from build123d import *

# Parameters (mm, degrees)
SKETCH1_W           = 19.8
SKETCH1_H           = 25
SKETCH1_R           = 1.15
BOSS_EXTRUDE1_DEPTH = 3
SKETCH2_W           = 19.8
SKETCH2_H           = 3
BOSS_EXTRUDE2_DEPTH = 26
CHAMFER1_SIZE       = 3
CUT_EXTRUDE1_DEPTH  = 15
CHAMFER2_SIZE       = 4
FILLET2_R           = 0.5


with BuildPart() as part:
    # Sketch1 → Boss-Extrude1 (new body)
    with BuildSketch(Plane.XY):
        with Locations((0, 1.287671233)):
            Rectangle(SKETCH1_W, SKETCH1_H)
        with Locations((-4.75, 10.787671233)):
            Circle(SKETCH1_R, mode=Mode.SUBTRACT)
        with Locations(Location((4.75, 10.787671233, 0), (0, 0, 180))):
            Circle(SKETCH1_R, mode=Mode.SUBTRACT)
    extrude(amount=BOSS_EXTRUDE1_DEPTH)

    # Sketch2 → Boss-Extrude2 (add)
    with BuildSketch(Plane.XY.offset(3)):
        with Locations((0, -9.712328767)):
            Rectangle(SKETCH2_W, SKETCH2_H)
    extrude(amount=BOSS_EXTRUDE2_DEPTH)

    # Chamfer1
    chamfer1_edges = [part.edges().sort_by_distance(p)[0] for p in [
        (0, -8.212328767, 3),
        (-9.9, 13.787671233, 1.5),
        (9.9, 13.787671233, 1.5),
    ]]
    chamfer(chamfer1_edges, length=CHAMFER1_SIZE)

    # Sketch4 → Cut-Extrude1 (cut)
    with BuildSketch(Plane(origin=(0, -8.212328767, 0), x_dir=(1, 0, 0), z_dir=(0, 1, 0))):
        with BuildLine():
            Line((2.647058824, -22.5), (2.647058824, -9.5))
            ThreePointArc((2.647058824, -9.5), (4.797058824, -7.35), (6.947058824, -9.5))
            Line((6.947058824, -9.5), (6.947058824, -22.5))
            ThreePointArc((6.947058824, -22.5), (4.797058824, -24.65), (2.647058824, -22.5))
        make_face()
        with BuildLine():
            Line((-2.647058824, -22.5), (-2.647058824, -9.5))
            ThreePointArc((-2.647058824, -9.5), (-4.797058824, -7.35), (-6.947058824, -9.5))
            Line((-6.947058824, -9.5), (-6.947058824, -22.5))
            ThreePointArc((-6.947058824, -22.5), (-4.797058824, -24.65), (-2.647058824, -22.5))
        make_face()
    extrude(amount=-CUT_EXTRUDE1_DEPTH, mode=Mode.SUBTRACT)

    # Chamfer2
    chamfer2_edges = [part.edges().sort_by_distance(p)[0] for p in [
        (-9.9, -9.712328767, 29),
        (9.9, -9.712328767, 29),
    ]]
    chamfer(chamfer2_edges, length=CHAMFER2_SIZE)

    # Fillet2
    fillet2_edges = [part.edges().sort_by_distance(p)[0] for p in [
        (-5.9, 10.787671233, 0),
        (5.9, 10.787671233, 0),
        (0, 13.787671233, 0),
        (0, 13.787671233, 3),
        (-6.9, 13.787671233, 1.5),
        (6.9, 13.787671233, 1.5),
        (-9.9, -0.212328767, 0),
        (-8.4, 12.287671233, 0),
        (8.4, 12.287671233, 0),
        (9.9, 2.787671233, 3),
        (9.9, 10.787671233, 1.5),
        (-9.9, 2.787671233, 3),
        (-8.4, 12.287671233, 3),
        (8.4, 12.287671233, 3),
        (-9.9, 10.787671233, 1.5),
        (-9.9, -6.712328767, 4.5),
        (9.9, -6.712328767, 4.5),
        (0, -11.212328767, 0),
        (9.9, -0.212328767, 0),
        (-5.9, -9.712328767, 29),
        (5.9, -9.712328767, 29),
        (9.9, -8.212328767, 15.5),
        (-9.9, -8.212328767, 15.5),
        (9.9, -11.212328767, 12.5),
        (9.9, -9.712328767, 25),
        (-9.9, -11.212328767, 12.5),
        (-9.9, -9.712328767, 25),
    ]]
    fillet(fillet2_edges, radius=FILLET2_R)


solid = part.part
The listing builds one solid part. Answer for the finished solid, in the listing's coordinates (mm). A direction names the side the tool comes from. Give positions to 0.01 mm unless a question says otherwise; leave off trailing zeros. Write each loop counter-clockwise with the first axis right and the second up, starting at its lowest first coordinate (ties: lowest second). Pieces come first, ordered by that corner, then holes. Notation, with made-up numbers: (-36.5, -2) -> (5.5, -2) arc R18 cw to (5.5, 18) -> close; hole circle Ø4 at (-19.75, -20.5). An arc over 180 degrees is marked (long way). Use a Markdown table: item, result.
(1) Determine the mould class of faces 1 (the flat face through (-2.647, -10, 16)), 2 (the flat face through (0, 13.788, 1)), 3 (the flat face through (-7.9, -9.7, 27)), 4 (the cylindrical face through (-4.84, -9.69, 24.65)) for opening direction Z: released by +Z, released by -Z, zero draft, split by the parting line, or undercut.
Return value:
| item | result |
|---|---|
| face 1 | undercut |
| face 2 | zero draft |
| face 3 | released by +Z |
| face 4 | undercut |
(2) Section B-B, the plane z = 15.75 is taken. Determine the outline of the cut face in (x, y), then the cut area to 3 significant figures.
Return value:
| item | result |
|---|---|
| outline | (-9.9, -10.71) arc R0.5 ccw to (-9.4, -11.21) -> (-6.95, -11.21) -> (-6.95, -8.21) -> (-9.4, -8.21) arc R0.5 ccw to (-9.9, -8.71) -> close; (-2.65, -11.21) -> (2.65, -11.21) -> (2.65, -8.21) -> (-2.65, -8.21) -> close; (6.95, -11.21) -> (9.4, -11.21) arc R0.5 ccw to (9.9, -10.71) -> (9.9, -8.71) arc R0.5 ccw to (9.4, -8.21) -> (6.95, -8.21) -> close |
| area | 33.4 mm2 |
(3) Section D-D, the plane x = -4.75 is taken. Determine the outline of the cut face in (y, z), then the cut area to 3 significant figures.
Return value:
| item | result |
|---|---|
| outline | (-11.21, 0.5) arc R0.5 ccw to (-10.71, 0) -> (9.14, 0) arc R0.5 ccw to (9.64, 0.5) -> (9.64, 3) -> (-5.21, 3) -> (-8.21, 6) -> (-8.21, 7.35) -> (-11.21, 7.35) -> close; (-11.21, 24.65) -> (-8.21, 24.65) -> (-8.21, 29) -> (-11.21, 29) -> close; (11.94, 0.5) arc R0.5 ccw to (12.44, 0) -> (13.29, 0) arc R0.5 ccw to (13.79, 0.5) -> (13.79, 2.5) arc R0.5 ccw to (13.29, 3) -> (11.94, 3) -> close |
| area | 98.4 mm2 |
(4) Find the intervals of material crossed by probe 1 along Y at (x, z) = (4.75, 1.1); probe 2 along Z at (x, y) = (5.75, -4); probe 3 along Z at (x, y) = (-6.75, -8.75), in increasing order. Write a range as from..to.
Return value:
| item | result |
|---|---|
| probe 1 | -11.21..9.64, 11.94..13.79 |
| probe 2 | 0..3 |
| probe 3 | 0..8.6, 23.4..28.15 |
(5) Flat-ended cylindrical pins translate along their axes: P1, Ø1.5, axis at x = 0.5, z = 4.5, coming from the +Y side; P2, Ø2, axis at x = -7, y = 4.5, coming from the +Z side; P3, Ø10, axis at x = -0.5, z = 9, coming from the +Y side. Find the tip coordinate at first contact, or state that the pin passes through.
Return value:
| item | result |
|---|---|
| P1 | y = -5.96 |
| P2 | z = 3 |
| P3 | y = -6.21 |
(6) For faces 5 (the cylindrical face through (-9.757, -6.842, 4.417)), 6 (the flat face through (-6.947, -10, 16)), 7 (the flat face through (0, -8.212, 17)), determine the directions among +Z, -Z, +X, -X, +Y, -Y from which every point of the face is accessible in a straight line to the end or side of a thin tool.
Return value:
| item | result |
|---|---|
| face 5 | +Z, -X, +Y |
| face 6 | +Y, -Y |
| face 7 | +Z, +X, -X, +Y |
(7) Section C-C, the plane y = 0.5 is taken. Determine the outline of the cut face in (x, z), then the cut area to 3 significant figures.
Return value:
| item | result |
|---|---|
| outline | (-9.9, 0.5) arc R0.5 ccw to (-9.4, 0) -> (9.4, 0) arc R0.5 ccw to (9.9, 0.5) -> (9.9, 2.5) arc R0.5 ccw to (9.4, 3) -> (-9.4, 3) arc R0.5 ccw to (-9.9, 2.5) -> close |
| area | 59.2 mm2 |
(8) Section A-A, the plane x = -0.25 is taken. Determine the outline of the cut face in (y, z).
Return value:
| item | result |
|---|---|
| outline | (-11.21, 0.5) arc R0.5 ccw to (-10.71, 0) -> (13.29, 0) arc R0.5 ccw to (13.79, 0.5) -> (13.79, 2.5) arc R0.5 ccw to (13.29, 3) -> (-5.21, 3) -> (-8.21, 6) -> (-8.21, 29) -> (-11.21, 29) -> close |
